Could you check a few things on this drawing? It's one solid part, dimensions in mm from its lowest x, y, z. A direction names the side the tool comes from. Give positions to 0.01 mm unless a question says otherwise; leave off trailing zeros. Order: outer loops, then holes, each group sorted by start corner. A loop starts at its lowest first (then second) coordinate and runs counter-clockwise, first axis right, second up.
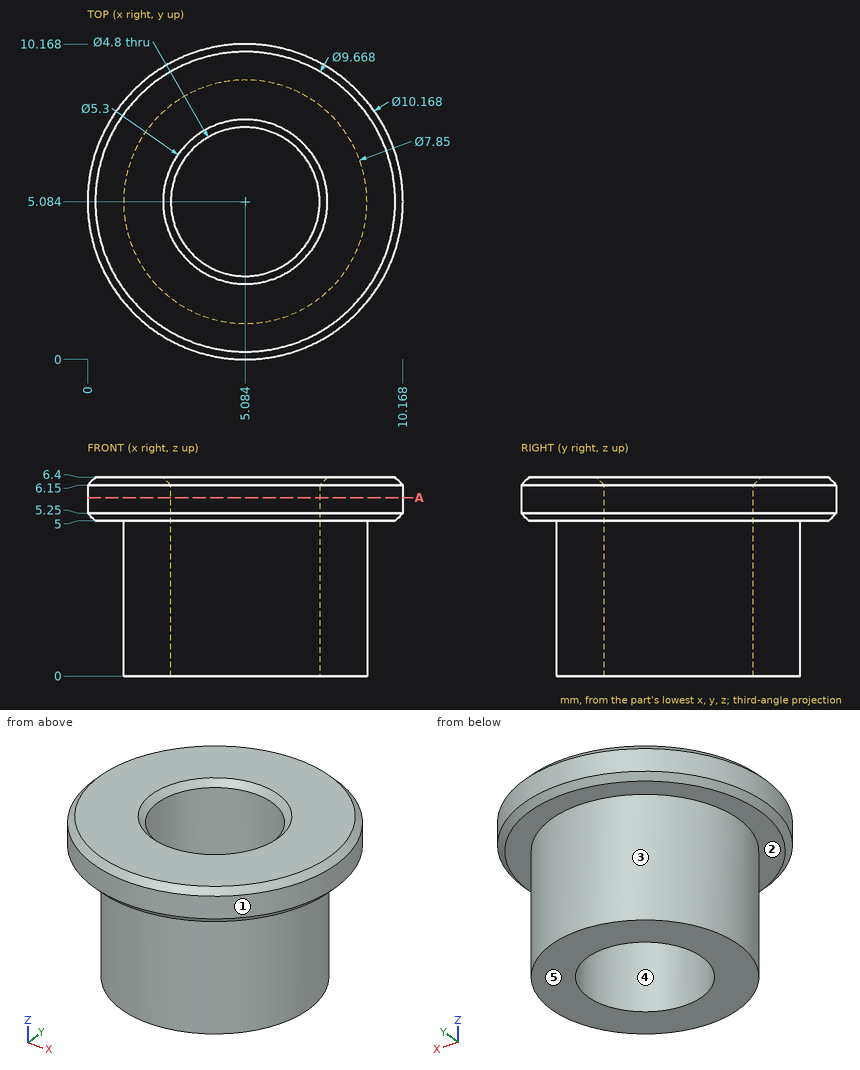
Item 1: We'd pull the mould along X, two halves only. Please class the marked faces 3, 4 and 5: +X half, -X half, draft (parallel to the pull), parting line (faces both ways), or undercut.
Findings:
face 3: parting line
face 4: undercut
face 5: draft
Item 2: For pin 1 (1 mm diameter, centred on y = 5, z = 3.5, fed in from -X); pin 2 (1.5 mm diameter, centred on x = 2, y = 9, fed in from -Z), each with a flat end and sliding along its axis, tell me the tip position at first contact or that it passes through.
Findings:
pin 1: stops at x = 1.16
pin 2: stops at z = 5
Item 3: Imagine slicing it at A-A on z = 5.75. List the corners of the cut face in (x, y) for me.
Findings:
outline: circle Ø10.17 at (5.08, 5.08); hole circle Ø4.8 at (5.08, 5.08)
Item 4: Please list where these lines run through material, in increasing order: line 1 along Y through (x, z) = (5, 0.75) (1 decimal); line 2 along Z through (x, y) = (7.75, 2).
Findings:
line 1: y = 1.2 to 2.7, 7.5 to 9
line 2: z = 5 to 6.4
Item 5: For the marked faces 1 and 2, which set-ups out of +Z, -Z, +X, -X, +Y, -Y let a thin tool reach every point of the face, with its end or its side?
Findings:
face 1: +Z, -Z
face 2: -Z
